```python
from build123d import *

# Parameters (mm, degrees)
BOSS_EXTRUDE1_DEPTH = 58.42
FILLET9_START       = -1
FILLET9_DEPTH       = 60
FILLET9_2_DEPTH     = 58.42


with BuildPart() as part:
    # Sketch1 → Boss-Extrude1 (new body)
    with BuildSketch(Plane(origin=(0, 0, 0), x_dir=(1, 0, 0), z_dir=(0, 1, 0))):
        with BuildLine():
            Line((-66.673768512, 0), (-37.067821873, 47.633329988))
            ThreePointArc((-37.067821873, 47.633329988), (-11.329209284, 68.541566023), (21.82652777, 69.113940477))
            Line((21.82652777, 69.113940477), (53.138492197, 58.903517294))
            Line((53.138492197, 58.903517294), (0, -77.45185891))
            Line((0, -77.45185891), (-66.673768512, -77.45185891))
            Line((-66.673768512, -77.45185891), (-66.673768512, 0))
        make_face()
    extrude(amount=BOSS_EXTRUDE1_DEPTH)

    # Fillet9: read off the stored shape, not the designer's step
    # Fillet9 outline → Fillet9 (cut)
    with BuildSketch(Plane(origin=(0, 0, 0), x_dir=(1, 0, 0), z_dir=(0, 1, 0)).offset(FILLET9_START)):
        with BuildLine():
            Line((53.138492197, 58.903517294), (42.560128995, 62.352983555))
            add(Edge.make_bspline(
                [(42.560128995, 62.352983555), (45.276451429, 55.785497085), (45.88017533, 47.021967979), (44.583604834, 36.951353495), (41.094604397, 27.998446712), (37.605603959, 19.045539929)],
                knots=[0.582099673, 0.582099673, 0.582099673, 0.582099673, 0.582099673, 0.582099673, 1, 1, 1, 1, 1, 1], degree=5))
            Line((37.605603959, 19.045539929), (53.138492197, 58.903517294))
        make_face()
    extrude(amount=FILLET9_DEPTH, mode=Mode.SUBTRACT)

    # Fillet9 2 outline → Fillet9 2 (add)
    with BuildSketch(Plane(origin=(0, 0, 0), x_dir=(1, 0, 0), z_dir=(0, 1, 0))):
        with BuildLine():
            add(Edge.make_bspline(
                [(-9.808315325, 69.069133652), (-0.482865879, 72.139293798), (12.240866744, 73.831219733), (27.210316696, 75.821767739), (36.460068296, 72.746962644), (41.411307971, 64.848690609), (42.026486953, 63.643215838), (42.560128995, 62.352983555)],
                knots=[0, 0, 0, 0, 0, 0, 0.5, 0.5, 0.582099673, 0.582099673, 0.582099673, 0.582099673, 0.582099673, 0.582099673], degree=5))
            ThreePointArc((-9.808315325, 69.069133652), (6.005529482, 71.616813676), (21.82652777, 69.113940477))
            Line((21.82652777, 69.113940477), (42.560128995, 62.352983555))
        make_face()
    extrude(amount=FILLET9_2_DEPTH)


solid = part.part
```
Work out the finished part from the listing and answer in its coordinate system (mm). Give positions to 0.01 mm unless a question says otherwise; leave off trailing zeros. Loops run counter-clockwise (first coordinate to the right, second up) from the corner with the lowest first, then second, coordinate; pieces in that order, holes last. Notation, with made-up numbers: (79.5, 22.25) -> (125.5, 22.25) arc R23 ccw to (125.5, 32.25) -> close; hole circle Ø7 at (22.5, 16). An arc over 180 degrees is marked (long way). Put each result on its own line as item: value. Start each with the question number.
Item 1: The part is cut by section A-A (z = 67.5). Give the vertices of the cut face in (x, y).
Item 2: The part is cut by section B-B (x = -15). Give the vertices of the cut face in (y, z), then the cut area to 3 significant figures.
Item 3: Find the intervals of material crossed by L1, parallel to X at y = 42, z = -32.5; L2, parallel to X at y = 39, z = 35.5; L3, parallel to Z at x = -1, y = 30, in increasing order. Write a range as [from, to].
Item 4: Each of these flat-tipped pins is pushed along its axis until it touches: P1, Ø8, axis at y = 32, z = -9, coming from the +X side; P2, Ø1, axis at x = 15, z = -52.5, coming from the -Y side; P3, Ø5, axis at x = -53.5, y = 8.5, coming from the -Z side; P4, Ø12, axis at x = -37, y = 23, coming from the -Z side. Where does it stop, or does it pass through?
Answers below:
1. outline: (-66.67, 0) -> (3.88, 0) -> (3.88, 58.42) -> (-66.67, 58.42) -> close
2. outline: (0, -67.04) -> (58.42, -67.04) -> (58.42, 77.45) -> (0, 77.45) -> close
2. area: 8,440 mm2
3. L1: [-46.47, 42.3]
3. L2: [-66.67, 16.35]
3. L3: [-71.34, 77.45]
4. P1: x = 35.25
4. P2: y = 0
4. P3: z = -25.22
4. P4: z = -55.54
